```python
from build123d import *

# Parameters (mm, degrees)
SKETCH1_W                = 5.5
SKETCH1_H                = 41.9
BOSS_EXTRUDE1_DEPTH      = 4
BOSS_EXTRUDE1_DEPTH_BACK = 4
BOSS_EXTRUDE2_DEPTH      = 3.2
BOSS_EXTRUDE2_DEPTH_BACK = 3.2
CUT_EXTRUDE1_DEPTH       = 13.2
CUT_EXTRUDE1_DEPTH_BACK  = 13.2
BOSS_EXTRUDE3_DEPTH      = 2.85
BOSS_EXTRUDE3_DEPTH_BACK = 2.85
BOSS_EXTRUDE4_DEPTH      = 2.85
BOSS_EXTRUDE4_DEPTH_BACK = 2.85
CUT_EXTRUDE2_DEPTH       = 4
CUT_EXTRUDE3_DEPTH       = 1.5
CUT_EXTRUDE3_DEPTH_BACK  = 1.5
CUT_EXTRUDE4_DEPTH       = 1.5
CUT_EXTRUDE4_DEPTH_BACK  = 1.5


with BuildPart() as part:
    # Sketch1 → Boss-Extrude1 (new body, two sides)
    with BuildSketch(Plane(origin=(0, 0, 0), x_dir=(0, 0, -1), z_dir=(1, 0, 0))) as boss_extrude1_sk:
        with Locations((2.75, 15.05)):
            Rectangle(SKETCH1_W, SKETCH1_H)
    extrude(amount=BOSS_EXTRUDE1_DEPTH)
    extrude(boss_extrude1_sk.sketch, amount=-BOSS_EXTRUDE1_DEPTH_BACK)

    # Sketch2 → Boss-Extrude2 (add, two sides)
    with BuildSketch(Plane(origin=(0, 0, 0), x_dir=(0, 0, -1), z_dir=(1, 0, 0))) as boss_extrude2_sk:
        with BuildLine():
            Line((-3.3, 34.5), (-0.3, 34.5))
            ThreePointArc((-0.3, 34.5), (-0.087867966, 34.412132034), (0, 34.2))
            Line((0, 34.2), (0, 36))
            Line((0, 36), (-3.3, 36))
            Line((-3.3, 36), (-3.3, 34.5))
        make_face()
    extrude(amount=BOSS_EXTRUDE2_DEPTH)
    extrude(boss_extrude2_sk.sketch, amount=-BOSS_EXTRUDE2_DEPTH_BACK)

    # Sketch3 → Cut-Revolve1 (revolve, cut)
    with BuildSketch(Plane(origin=(0, 0, 0), x_dir=(0, 0, -1), z_dir=(1, 0, 0))):
        Polygon((0, 30), (0, 31.5), (2.4, 31.5), (2.4, 33), (5.5, 33), (5.5, 30), align=None)
    revolve(axis=Axis((0, 30, -5.5), (0, 0, 1)), mode=Mode.SUBTRACT)

    # Sketch4 → Cut-Revolve2 (revolve, cut)
    with BuildSketch(Plane(origin=(0, 0, 0), x_dir=(0, 0, -1), z_dir=(1, 0, 0))):
        Polygon((0, 0), (0, 1.5), (2.4, 1.5), (2.4, 3), (5.5, 3), (5.5, 0), align=None)
    revolve(axis=Axis((0, 0, -5.5), (0, 0, 1)), mode=Mode.SUBTRACT)

    # Sketch5 → Cut-Extrude1 (cut, two sides)
    with BuildSketch(Plane(origin=(0, 15, 0), x_dir=(1, 0, 0), z_dir=(0, 1, 0))) as cut_extrude1_sk:
        with BuildLine():
            Line((-3.5, -2.4), (3.5, -2.4))
            Line((3.5, -2.4), (3.5, 0))
            Line((3.5, 0), (2.787070261, 0))
            ThreePointArc((2.787070261, 0), (2.249770652, 0.156608554), (1.880762474, 0.577381738))
            Line((1.880762474, 0.577381738), (1.327022899, 1.764880088))
            ThreePointArc((1.327022899, 1.764880088), (0.921113903, 2.22773059), (0.330084334, 2.4))
            Line((0.330084334, 2.4), (-0.330084334, 2.4))
            ThreePointArc((-0.330084334, 2.4), (-0.921113903, 2.22773059), (-1.327022899, 1.764880088))
            Line((-1.327022899, 1.764880088), (-1.880762474, 0.577381738))
            ThreePointArc((-1.880762474, 0.577381738), (-2.249770652, 0.156608554), (-2.787070261, 0))
            Line((-2.787070261, 0), (-3.5, 0))
            Line((-3.5, 0), (-3.5, -2.4))
        make_face()
    extrude(amount=CUT_EXTRUDE1_DEPTH, mode=Mode.SUBTRACT)
    extrude(cut_extrude1_sk.sketch, amount=-CUT_EXTRUDE1_DEPTH_BACK, mode=Mode.SUBTRACT)

    # Sketch6 → Boss-Extrude3 (add, two sides)
    with BuildSketch(Plane(origin=(0, 0, 0), x_dir=(0, 0, -1), z_dir=(1, 0, 0))) as boss_extrude3_sk:
        with BuildLine():
            Line((0, 1.626838695), (2.4, 1.626838695))
            Line((2.4, 1.626838695), (2.4, 5.797156532))
            ThreePointArc((2.4, 5.797156532), (2.294462086, 5.198621281), (1.990577775, 4.672278215))
            Line((1.990577775, 4.672278215), (0.304142224, 2.662462588))
            ThreePointArc((0.304142224, 2.662462588), (0.078399593, 2.271464882), (0, 1.826838695))
            Line((0, 1.826838695), (0, 1.626838695))
        make_face()
    extrude(amount=BOSS_EXTRUDE3_DEPTH)
    extrude(boss_extrude3_sk.sketch, amount=-BOSS_EXTRUDE3_DEPTH_BACK)

    # Sketch7 → Boss-Extrude4 (add, two sides)
    with BuildSketch(Plane(origin=(0, 0, 0), x_dir=(0, 0, -1), z_dir=(1, 0, 0))) as boss_extrude4_sk:
        with BuildLine():
            Line((0, 28.373161305), (0, 28.173161305))
            ThreePointArc((0, 28.173161305), (0.078399593, 27.728535118), (0.304142224, 27.337537412))
            Line((0.304142224, 27.337537412), (1.990577775, 25.327721785))
            ThreePointArc((1.990577775, 25.327721785), (2.294462086, 24.801378719), (2.4, 24.202843468))
            Line((2.4, 24.202843468), (2.4, 28.373161305))
            Line((2.4, 28.373161305), (0, 28.373161305))
        make_face()
    extrude(amount=BOSS_EXTRUDE4_DEPTH)
    extrude(boss_extrude4_sk.sketch, amount=-BOSS_EXTRUDE4_DEPTH_BACK)

    # Sketch8 → Cut-Extrude2 (cut)
    with BuildSketch(Plane.XY):
        Polygon((-15, -15.264317181), (16.073788546, -15.264317181), (16.073788546, -1.569872981), (4.4, -1.569872981), (1.9, -5.9), (-1.9, -5.9), (-4.4, -1.569872981), (-15, -1.569872981), align=None)
    extrude(amount=-CUT_EXTRUDE2_DEPTH, mode=Mode.SUBTRACT)

    # Sketch9 → Revolve1 (revolve)
    with BuildSketch(Plane(origin=(0, 0, 0), x_dir=(0, 0, -1), z_dir=(1, 0, 0))):
        Polygon((-34.5, 30), (-34.5, 31.1935), (-34.1935, 31.5), (-24.8065, 31.5), (-24.5, 31.1935), (2.4, 31.1935), (2.4, 32.6), (4.5, 32.6), (4.5, 30), align=None)
    revolve(axis=Axis((0, 30, -4.5), (0, 0, 1)))

    # Sketch10 → Revolve2 (revolve)
    with BuildSketch(Plane(origin=(0, 0, 0), x_dir=(0, 0, -1), z_dir=(1, 0, 0))):
        Polygon((-34.5, 0), (-34.5, 1.1935), (-34.1935, 1.5), (-24.8065, 1.5), (-24.5, 1.1935), (2.4, 1.1935), (2.4, 2.6), (4.5, 2.6), (4.5, 0), align=None)
    revolve(axis=Axis((0, 0, -4.5), (0, 0, 1)))

    # Sketch11 → Cut-Extrude3 (cut, two sides)
    with BuildSketch(Plane(origin=(0, 0, -4.5), x_dir=(-1, 0, 0), z_dir=(0, 0, -1))) as cut_extrude3_sk:
        Polygon((0.5, 28), (0.5, 29.5), (2, 29.5), (2, 30.5), (0.5, 30.5), (0.5, 32), (-0.5, 32), (-0.5, 30.5), (-2, 30.5), (-2, 29.5), (-0.5, 29.5), (-0.5, 28), align=None)
    extrude(amount=CUT_EXTRUDE3_DEPTH, mode=Mode.SUBTRACT)
    extrude(cut_extrude3_sk.sketch, amount=-CUT_EXTRUDE3_DEPTH_BACK, mode=Mode.SUBTRACT)

    # Sketch12 → Cut-Extrude4 (cut, two sides)
    with BuildSketch(Plane(origin=(0, 0, -4.5), x_dir=(-1, 0, 0), z_dir=(0, 0, -1))) as cut_extrude4_sk:
        Polygon((0.5, -2), (0.5, -0.5), (2, -0.5), (2, 0.5), (0.5, 0.5), (0.5, 2), (-0.5, 2), (-0.5, 0.5), (-2, 0.5), (-2, -0.5), (-0.5, -0.5), (-0.5, -2), align=None)
    extrude(amount=CUT_EXTRUDE4_DEPTH, mode=Mode.SUBTRACT)
    extrude(cut_extrude4_sk.sketch, amount=-CUT_EXTRUDE4_DEPTH_BACK, mode=Mode.SUBTRACT)


solid = part.part
```
Geometry: final body of the model. Coordinates: model frame, mm. A direction names the side the tool comes from. Round coordinates to 2 decimals unless told otherwise and drop trailing zeros. Order: outer loops, then holes, each group sorted by start corner. A loop starts at its lowest first (then second) coordinate and runs counter-clockwise, first axis right, second up. Notation, with made-up numbers: M 36.5,-12 L 65.5,-12 A16 ccw 65.5,-6 Z; hole C -20.75,14 d2. An arc over 180 degrees is marked long. One line per item, written item: value.
(1) Pull-direction query (Y, two-part tool) for faces 4 (the flat face through (-2, 0, -4)), 5 (the flat face through (-4, 15, -3)); classes: pulls with the +Y half, pulls with the -Y half, needs draft (parallel to the pull), parting line crosses it, or undercut.
Result sheet:
face 4: undercut
face 5: needs draft
(2) Reachability of faces 1 (the cylindrical face through (1.165, -0.259, 10.862)), 2 (the flat face through (-1.6, 14.83, -1.18)), 3 (the flat face through (-1, 29.5, -4)) from +Z, -Z, +X, -X, +Y, -Y: full face, straight path, thin tool, end or side. Return the list, or none.
Result sheet:
face 1: none
face 2: +Z
face 3: -Z
(3) Cut plane B-B (z = 12.5). Return the cut outline in (x, y), and give its area (3 significant figures).
Result sheet:
outline: C 0,0 d2.39; C 0,30 d2.39
area: 8.95 mm2
(4) Cut plane D-D (z = 25.5). Return the cut outline in (x, y).
Result sheet:
outline: C 0,0 d3; C 0,30 d3
(5) Cut plane C-C (y = 18.5). Return the cut outline in (x, z), and give its area (3 significant figures).
Result sheet:
outline: M -4,-5.5 L 4,-5.5 L 4,0 L 2.79,0 A1 ccw 1.88,-0.58 L 1.33,-1.76 A1.1 cw 0.33,-2.4 L -0.33,-2.4 A1.1 cw -1.33,-1.76 L -1.88,-0.58 A1 ccw -2.79,0 L -4,0 Z
area: 36.4 mm2
(6) Line query: probe 1 along X at (y, z) = (30, -3.8); probe 2 along X at (y, z) = (0, -1); probe 3 along Y at (x, z) = (0, -4.9). Output: solid intervals per line, ascending. Write a range as [from, to].
Result sheet:
probe 1: [-4, -3], [-2.6, -2], [2, 2.6], [3, 4]
probe 2: [-4, -1.5], [-1.19, 1.19], [1.5, 4]
probe 3: [-5.9, -3], [3, 27], [33, 36]
(7) Pin query (flat end, axial travel): P1, Ø3, axis at x = -1, y = 7.5, coming from the +Z side; P2, Ø10, axis at y = 25.5, z = 18, coming from the -X side; P3, Ø10, axis at y = 7.5, z = 10, coming from the -X side; P4, Ø0.9, axis at y = 35.5, z = 1, coming from the +X side. Return the tip coordinate at first contact, or that it passes through.
Result sheet:
P1: z = -0.04
P2: x = -1.19
P3: through
P4: x = 3.2
